```python
from build123d import *

# Parameters (mm, degrees)
RESSALTO_EXTRUS_O1_DEPTH = 10
RESSALTO_EXTRUS_O2_DEPTH = 10
ESBO_O3_R                = 12
CORTE_EXTRUS_O1_DEPTH    = 21


with BuildPart() as part:
    # Esboço1 → Ressalto-extrusão1 (new body)
    with BuildSketch(Plane.XY):
        with BuildLine():
            Line((0, 26), (80, 26))
            ThreePointArc((80, 26), (106, 0), (80, -26))
            Line((80, -26), (0, -26))
            ThreePointArc((0, -26), (-26, 0), (0, 26))
        make_face()
    extrude(amount=RESSALTO_EXTRUS_O1_DEPTH)

    # Esboço2 → Ressalto-extrusão2 (add)
    with BuildSketch(Plane.XY.offset(10)):
        with BuildLine():
            Line((0, 13), (57.483339502, 13))
            ThreePointArc((57.483339502, 13), (106, 0), (57.483339502, -13))
            Line((57.483339502, -13), (0, -13))
            ThreePointArc((0, -13), (-13, 0), (0, 13))
        make_face()
    extrude(amount=RESSALTO_EXTRUS_O2_DEPTH)

    # Esboço3 → Corte-extrusão1 (cut, through all)
    with BuildSketch(Plane.XY.offset(20)):
        with Locations((80, 0)):
            Circle(ESBO_O3_R)
        with BuildLine():
            Line((0, 7), (40, 7))
            ThreePointArc((40, 7), (47, 0), (40, -7))
            Line((40, -7), (0, -7))
            ThreePointArc((0, -7), (-7, 0), (0, 7))
        make_face()
    extrude(amount=-CORTE_EXTRUS_O1_DEPTH, mode=Mode.SUBTRACT)


solid = part.part
```
Part model, mm, in its own coordinate system. A direction names the side the tool comes from. Round coordinates to 2 decimals unless told otherwise and drop trailing zeros. Loops run counter-clockwise (first coordinate to the right, second up) from the corner with the lowest first, then second, coordinate; pieces in that order, holes last.
Item 1: Cut at D-D, the plane y = 0. Give the cut face in (x, z), then the cut area to 3 significant figures.
Item 2: 3-axis set-ups, long thin cutter, end or side, ignore diameter. For faces 1 (the face through (28, 13, 15)), 2 (the face through (20, -7, 10)), 3 (the face through (29, -13, 15)): which of +Z, -Z, +X, -X, +Y, -Y reach the whole face in a straight line?
Item 3: Cut at B-B, the plane z = 16. Give the cut face in (x, y), then the cut area to 3 significant figures.
Item 4: Mould opens along X. For faces 4 (the face through (47, 0, 10)), 5 (the face through (-13, 0, 15)), 6 (the face through (39, 26, 5)) say: +X half, -X half, draft (parallel to the pull), parting line (faces both ways), or undercut.
Item 5: Cut at C-C, the plane y = -9. Give the cut face in (x, z).
Item 6: Drill centre lines: line 1 (Y direction, x = 80, z = 5.5); line 2 (Z direction, x = 23, y = -14.5); line 3 (X direction, y = 4.5, z = 13.5). Where is each one in solid material? Low to high.
Item 7: Drop flat-ended pins along their axis: P1, Ø10, axis at y = -14, z = 15.5, coming from the -X side; P2, Ø6, axis at y = 0.5, z = 2.5, coming from the -X side; P3, Ø3, axis at y = 0.5, z = 13, coming from the -X side. Give the stop position or say it passes through.
Item 8: Cut at A-A, the plane x = 28. Give the cut face in (y, z).
A:
1. outline: (-26, 0) - (-7, 0) - (-7, 20) - (-13, 20) - (-13, 10) - (-26, 10) - close; (47, 0) - (68, 0) - (68, 20) - (47, 20) - close; (92, 0) - (106, 0) - (106, 20) - (92, 20) - close
1. area: 950 mm2
2. face 1: +Z, -X, +Y
2. face 2: +Z, -Z
2. face 3: +Z, -X, -Y
3. outline: (0, -13) - (57.48, -13) arc R26 ccw (long way) to (57.48, 13) - (0, 13) arc R13 ccw to start; hole (0, -7) - (40, -7) arc R7 ccw to (40, 7) - (0, 7) arc R7 ccw to start; hole circle Ø24 at (80, 0)
3. area: 2,660 mm2
4. face 4: undercut
4. face 5: -X half
4. face 6: draft
5. outline: (-24.39, 0) - (72.06, 0) - (72.06, 20) - (-9.38, 20) - (-9.38, 10) - (-24.39, 10) - close; (87.94, 0) - (104.39, 0) - (104.39, 20) - (87.94, 20) - close
6. line 1: y = -26 to -12, 12 to 26
6. line 2: z = 0 to 10
6. line 3: x = -12.2 to -5.36, 45.36 to 68.88, 91.12 to 105.61
7. P1: stops at x = -9.38
7. P2: stops at x = -26
7. P3: stops at x = -13
8. outline: (-26, 0) - (-7, 0) - (-7, 20) - (-13, 20) - (-13, 10) - (-26, 10) - close; (7, 0) - (26, 0) - (26, 10) - (13, 10) - (13, 20) - (7, 20) - close
